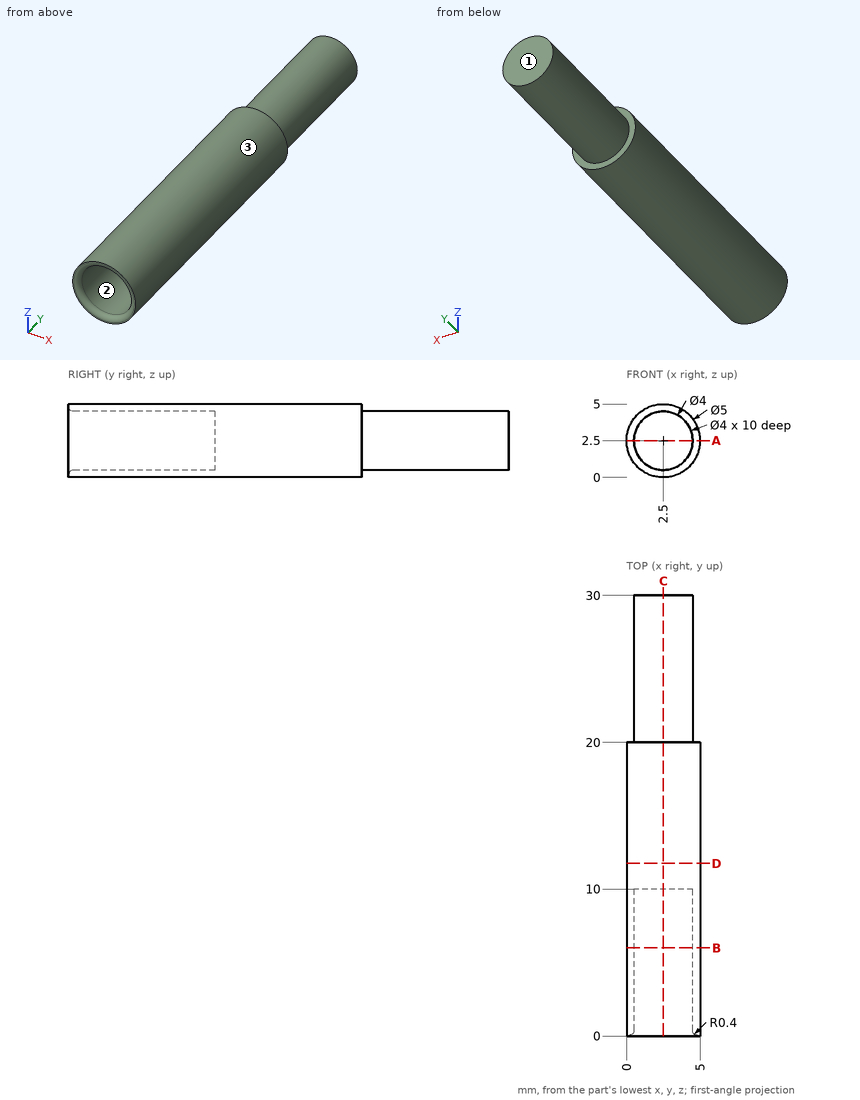
Geometry check sheet. Reference: drawing and pictorial views, mm from the part's lowest x, y, z. Coordinates: 2 decimals unless noted, no trailing zeros. Write each loop counter-clockwise with the first axis right and the second up, starting at its lowest first coordinate (ties: lowest second). Pieces come first, ordered by that corner, then holes. Notation, with made-up numbers: M -5,2.25 L 19,2.25 A15 cw 19,20.25 Z; hole C -14,82.25 d2. An arc over 180 degrees is marked long. Write item = value, one per line. Start each with the question number.
1. Mould release check, pull along Z, two halves, no side actions. Record for the marked faces 1, 2 and 3: pulls with the +Z half, pulls with the -Z half, needs draft (parallel to the pull), parting line crosses it, or undercut.
2. Sectioned sample at D-D (y = 11.75). Record the cut outline in (x, z).
3. Sectioned sample at C-C (x = 2.5). Record the cut outline in (y, z).
4. Go/stop test with flat-tipped pins: pin 1 (2 mm diameter, centred on x = 2.5, z = 2.5, fed in from -Y); pin 2 (1.5 mm diameter, centred on y = 10, z = 4.5, fed in from -X). Record where each tip stops, or that it passes through.
5. Thickness scan on probe 1 along Z at (x, y) = (2.5, 3.5); probe 2 along Y at (x, z) = (2.7, 2.4); probe 3 along Z at (x, y) = (2.4, 13). Record the ranges inside material, lowest first.
6. Sectioned sample at A-A (z = 2.5). Record the cut outline in (x, y).
7. Sectioned sample at B-B (y = 6). Record the cut outline in (x, z).
The answers:
q1.face_1 = needs draft
q1.face_2 = undercut
q1.face_3 = parting line crosses it
q2.outline = C 2.5,2.5 d5
q3.outline = M 0,0 L 20,0 L 20,0.5 L 30,0.5 L 30,4.5 L 20,4.5 L 20,5 L 0,5 L 0,4.9 A0.4 ccw 0.4,4.5 L 10,4.5 L 10,0.5 L 0.4,0.5 A0.4 ccw 0,0.1 Z
q4.pin_1 = 10
q4.pin_2 = 0.33
q5.probe_1 = 0 to 0.5, 4.5 to 5
q5.probe_2 = 10 to 30
q5.probe_3 = 0 to 5
q6.outline = M 0,0 L 0.1,0 A0.4 ccw 0.5,0.4 L 0.5,10 L 4.5,10 L 4.5,0.4 A0.4 ccw 4.9,0 L 5,0 L 5,20 L 4.5,20 L 4.5,30 L 0.5,30 L 0.5,20 L 0,20 Z
q7.outline = C 2.5,2.5 d5; hole C 2.5,2.5 d4
